Source: CAD feature listing. Evaluate the final solid. Frame: model axes, mm. A direction names the side the tool comes from. Give positions to 0.01 mm unless a question says otherwise; leave off trailing zeros. Order: outer loops, then holes, each group sorted by start corner. A loop starts at its lowest first (then second) coordinate and runs counter-clockwise, first axis right, second up. Notation, with made-up numbers: M -12.5,-0.5 L 28.5,-0.5 A34 cw 28.5,33.5 Z; hole C 0.5,-6 d2. An arc over 180 degrees is marked long. Answer in a Markdown table with one row per item. Add a question column.
(1) Section query D-D, the plane y = 5.5. Return loops of the section in (x, z) (3 decimals), plus the area to 3 significant figures.
(2) Section query B-B, the plane y = 0. Count the separate pieces of the cut face and the enclosed holes in it, plus the area to 3 significant figures.
(3) Section query A-A, the plane x = 14.5. Return loops of the section in (y, z) (1 decimal), plus the area to 3 significant figures.
(4) Pin query (flat end, axial travel): P1, Ø1.5, axis at x = -9.5, y = 1.5, coming from the +Z side (3 decimals); P2, Ø1.9, axis at x = -17, z = 24.5, coming from the -Y side; P3, Ø2, axis at y = -10.5, z = 15, coming from the +X side. Return the tip coordinate at first contact, or that it passes through.
(5) Set-up query: faces 1 (the face through (-15.919, 0.228, 38.923)), 2 (the face through (0, -11, 16)), 3 (the face through (-17.5, -5.5, 25.4)), 4 (the face through (-16, -10.35, 25)), 5 (the face through (-7.01, 0.15, 10.96)). Return all of +Z, -Z, +X, -X, +Y, -Y with unobstructed straight access to the full face (end or side cutting, diameter ignored); none if empty.
(6) Mould query, pull axis X, two halves, no side actions, for faces 6 (the face through (0, 11, 16)), 7 (the face through (44, 7.013, 5)), 8 (the face through (-17.529, -5.525, 31.706)). Classes: pulls with the +X half, pulls with the -X half, needs draft (parallel to the pull), parting line crosses it, or undercut.
(7) Material intervals for line 1 along Z through (x, y) = (-23.1, 0); line 2 along Y through (x, z) = (40.5, 6); line 3 along X through (y, z) = (-7, 27), sorted ascending.
from build123d import *

# Parameters (mm, degrees)
F1_DEPTH       = 9.525
F2_W           = 25.4
F2_H           = 28.575
F3_DEPTH       = 12.7
F4_W           = 6.35
F4_H           = 28.575
F5_DEPTH       = 25.4
F7_DEPTH       = 6.35
F8_R           = 3.429
F9_DEPTH       = 25.4
F11_DEPTH      = 25.4
F11_DEPTH_BACK = 25.4
F13_DEPTH      = 3.175


with BuildPart() as f1:
    # F0 (on Top) → F1 (new body)
    with BuildSketch(Plane.XY):
        Polygon((101.6, 14.2875), (0, 14.2875), (-25.4, 14.2875), (-25.4, -14.2875), (0, -14.2875), (101.6, -14.2875), align=None)
    extrude(amount=F1_DEPTH)

    # F2 (on face) → F3 (join)
    with BuildSketch(Plane.XY.offset(9.525)):
        with Locations((-12.7, 0)):
            Rectangle(F2_W, F2_H)
    extrude(amount=F3_DEPTH)

    # F4 (on face) → F5 (join)
    with BuildSketch(Plane.XY.offset(22.225)):
        with Locations((-22.225, 0)):
            Rectangle(F4_W, F4_H)
    extrude(amount=F5_DEPTH)

    # F6 (on face) → F7 (join)
    with BuildSketch(Plane.YZ.offset(-19.05)):
        with BuildLine():
            Line((10.3502472592, 17.0163675877), (10.3502472592, 28.575))
            ThreePointArc((10.3502472592, 28.575), (0, 38.9252472592), (-10.3502472592, 28.575))
            Line((-10.3502472592, 28.575), (-10.3502472592, 17.0163675877))
            Line((-10.3502472592, 17.0163675877), (10.3502472592, 17.0163675877))
        make_face()
        Polygon((7.3323484187, 28.575), (3.6661742094, 22.225), (-3.6661742094, 22.225), (-7.3323484187, 28.575), (-3.6661742094, 34.925), (3.6661742094, 34.925), align=None, mode=Mode.SUBTRACT)
    extrude(amount=F7_DEPTH)

    # F8 (on face) → F9 (cut)
    with BuildSketch(Plane.YZ.offset(-19.05)):
        with BuildLine():
            Line((-14.2875, 47.625), (-14.2875, 28.575))
            ThreePointArc((-14.2875, 28.575), (0, 42.8625), (14.2875, 28.575))
            Line((14.2875, 28.575), (14.2875, 47.625))
            Line((14.2875, 47.625), (-14.2875, 47.625))
        make_face()
        with Locations((0, 28.575)):
            Circle(F8_R)
    extrude(amount=-F9_DEPTH, mode=Mode.SUBTRACT)

    # F10 (on face) → F11 (cut, two sides)
    with BuildSketch(Plane.XY.offset(9.525)) as f11_sk:
        with BuildLine():
            Line((87.3125, 7.0132897794), (0, 7.0132897794))
            ThreePointArc((0, 7.0132897794), (-7.0132897794, 0), (0, -7.0132897794))
            Line((0, -7.0132897794), (87.3125, -7.0132897794))
            ThreePointArc((87.3125, -7.0132897794), (94.3257897794, 0), (87.3125, 7.0132897794))
        make_face()
        with BuildLine():
            Line((103.5399436951, 14.2875), (87.3125, 14.2875))
            ThreePointArc((87.3125, 14.2875), (101.6, 0), (87.3125, -14.2875))
            Line((87.3125, -14.2875), (103.5399436951, -17.2526948154))
            Line((103.5399436951, -17.2526948154), (103.5399436951, 14.2875))
        make_face()
    extrude(amount=-F11_DEPTH, mode=Mode.SUBTRACT)
    extrude(f11_sk.sketch, amount=F11_DEPTH_BACK, mode=Mode.SUBTRACT)

    # F12 (on face) → F13 (cut)
    with BuildSketch(Plane.YZ.offset(-19.05)):
        Polygon((3.6661742094, 22.225), (7.3323484187, 28.575), (3.6661742094, 34.925), (-3.6661742094, 34.925), (-7.3323484187, 28.575), (-3.6661742094, 22.225), align=None)
    extrude(amount=-F13_DEPTH, mode=Mode.SUBTRACT)


solid = f1.part
Values follow:
| question | item | result |
|---|---|---|
| 1 | outline | M -25.4,0 L -4.352,0 L -4.352,22.225 L -12.7,22.225 L -12.7,25.401 L -22.225,25.401 L -22.225,31.749 L -12.7,31.749 L -12.7,37.343 L -19.05,37.343 L -19.05,41.761 L -25.4,41.761 Z; M 91.664,0 L 100.499,0 L 100.499,9.525 L 91.664,9.525 Z |
| 1 | area | 712 mm² |
| 2 | separate pieces | 3 |
| 2 | enclosed holes | 0 |
| 2 | area | 572 mm² |
| 3 | outline | M -14.3,0 L -7,0 L -7,9.5 L -14.3,9.5 Z; M 7,0 L 14.3,0 L 14.3,9.5 L 7,9.5 Z |
| 3 | area | 139 mm² |
| 4 | P1 | stops at z = 22.225 |
| 4 | P2 | stops at y = -10.35 |
| 4 | P3 | stops at x = 0 |
| 5 | face 1 | +Z, +X |
| 5 | face 2 | +Z, +X, +Y, -Y |
| 5 | face 3 | +X |
| 5 | face 4 | +Z, +X, -Y |
| 5 | face 5 | +Z, -Z |
| 6 | face 6 | pulls with the +X half |
| 6 | face 7 | undercut |
| 6 | face 8 | needs draft |
| 7 | line 1 | z = 0 to 25.15, 32 to 42.86 |
| 7 | line 2 | y = -14.29 to -7.01, 7.01 to 14.29 |
| 7 | line 3 | x = -25.4 to -12.7 |
